```python
from build123d import *

# Parameters (mm, degrees)
BOX002_W        = 30
BOX002_H        = 11
BOX002_DEPTH    = 20
CHAMFER_SIZE    = 10
BOX_W           = 30
BOX_H           = 30
BOX_DEPTH       = 30
BOX001_W        = 11
BOX001_H        = 30
BOX001_DEPTH    = 20
CHAMFER001_SIZE = 10


with BuildPart() as chamfer_body:
    # Box002 → Box002 (new body)
    with BuildSketch(Plane(origin=(-15, -25, 10), x_dir=(1, 0, 0), z_dir=(0, 0, 1))):
        with Locations((15, 5.5)):
            Rectangle(BOX002_W, BOX002_H)
    extrude(amount=BOX002_DEPTH)

    # Chamfer
    chamfer_edges = [chamfer_body.edges().sort_by_distance(p)[0] for p in [
        (0, -25, 10),
    ]]
    chamfer(chamfer_edges, length=CHAMFER_SIZE)


with BuildPart() as cube:
    # Box → Box (new body)
    with BuildSketch(Plane(origin=(-15, -15, 0), x_dir=(1, 0, 0), z_dir=(0, 0, 1))):
        with Locations((15, 15)):
            Rectangle(BOX_W, BOX_H)
    extrude(amount=BOX_DEPTH)


with BuildPart() as fusion:
    # Box001 → Box001 (new body)
    with BuildSketch(Plane(origin=(-25, -15, 10), x_dir=(1, 0, 0), z_dir=(0, 0, 1))):
        with Locations((5.5, 15)):
            Rectangle(BOX001_W, BOX001_H)
    extrude(amount=BOX001_DEPTH)

    # Chamfer001
    chamfer001_edges = [fusion.edges().sort_by_distance(p)[0] for p in [
        (-25, 0, 10),
    ]]
    chamfer(chamfer001_edges, length=CHAMFER001_SIZE)

    # Fusion: union Chamfer body, Cube
    add(chamfer_body.part)
    add(cube.part)


solid = fusion.part
```
Model file for the job. Use its own axes, mm. A direction names the side the tool comes from. Coordinates: 2 decimals unless noted, no trailing zeros. Loops run counter-clockwise (first coordinate to the right, second up) from the corner with the lowest first, then second, coordinate; pieces in that order, holes last. Notation, with made-up numbers: (85.5, 42) - (132.5, 42) arc R22 cw to (132.5, 64) - close; hole circle Ø10 at (11.25, 64). An arc over 180 degrees is marked (long way). Answer as a JSON object with one key per item and string values. Group by question number.
(1) Cut at B-B (x = 0). Give the cut face in (y, z).
(2) Cut at A-A (z = 28). Give the cut face in (x, y), then the cut area to 3 significant figures.
(3) Probe line 1 along X through (y, z) = (-0.5, 4.75); line 2 along Z through (x, y) = (-19, -10). List the from-to ranges inside material, lowest first.
(4) Cut at C-C (y = -16.5). Give the cut face in (x, z).
(5) Tool access for faces 1 (the face through (0, -25, 25)), 2 (the face through (-15, -20, 22)), 3 (the face through (-15, 0, 5)), 4 (the face through (0, -15, 5)): list every direction of +Z, -Z, +X, -X, +Y, -Y with a clear straight run to the whole face (end or side of a thin tool).
(6) Flat gauge pins, fed straight in: pin 1 (5 mm diameter, centred on y = 4.5, z = 3, fed in from -X); pin 2 (4 mm diameter, centred on x = -10.5, y = 4.5, fed in from -Z); pin 3 (5 mm diameter, centred on x = 6.5, z = 6.5, fed in from -Y). Where does each tip first touch, or does it go through?
(7) Cut at D-D (x = -19.5). Give the cut face in (y, z).
Geometry says:
{
 "1": {"outline": "(-25, 20) - (-15, 10) - (-15, 0) - (15, 0) - (15, 30) - (-25, 30) - close"},
 "2": {"outline": "(-25, -15) - (-15, -15) - (-15, -25) - (15, -25) - (15, 15) - (-25, 15) - close", "area": "1,500 mm^2"},
 "3": {"line 1": "x = -15 to 15", "line 2": "z = 14 to 30"},
 "4": {"outline": "(-15, 11.5) - (15, 11.5) - (15, 30) - (-15, 30) - close"},
 "5": {"face 1": "+Z, -Z, +X, -X, -Y", "face 2": "+Z, -Z, -X, -Y", "face 3": "-Z, -X, +Y, -Y", "face 4": "-Z, +X, -X, -Y"},
 "6": {"pin 1": "stops at x = -15", "pin 2": "stops at z = 0", "pin 3": "stops at y = -15"},
 "7": {"outline": "(-15, 14.5) - (15, 14.5) - (15, 30) - (-15, 30) - close"}
}
